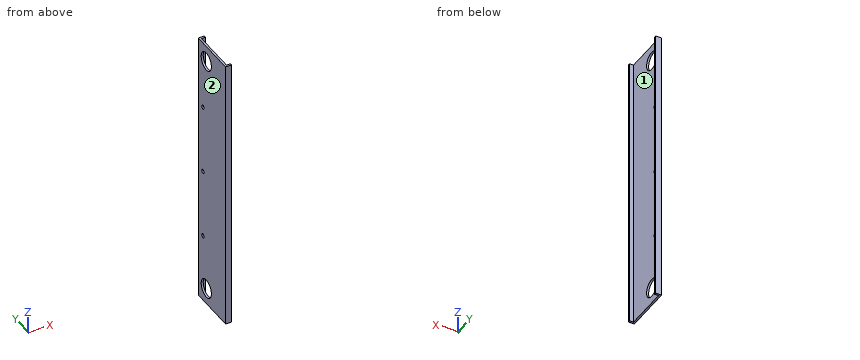
Autodesk Inventor part; units mm, degrees
ref_plane "YZ Plane" through (0, 0, 0) normal (1, 0, 0) x (0, 1, 0)
ref_plane "XZ Plane" through (0, 0, 0) normal (0, 1, 0) x (-1, 0, 0)
ref_plane "XY Plane" through (0, 0, 0) normal (0, 0, 1) x (1, 0, 0)
sketch "Sketch1" plane through (0, 0, 0) normal (0, 0, 1) x (1, 0, 0)
  line L0 (0, 0) -> (9.525, 0)
  line L1 (9.525, 76.2) -> (0, 76.2)
  line L2 (0, 76.2) -> (0, 0)
  line L3 (9.525, 3.175) -> (3.175, 3.175)
  line L4 (3.175, 3.175) -> (3.175, 73.025)
  line L5 (3.175, 73.025) -> (9.525, 73.025)
  line L6 (9.525, 0) -> (9.525, 3.175)
  line L7 (9.525, 73.025) -> (9.525, 76.2)
  dimension "d0" = 3.175
  dimension "d2" = 3.175
  dimension "d3" = 3.175
  dimension "d4" = 76.2
  dimension "d5" = 9.525
extrude "Extrusion1" add sketch "Sketch1" along normal blind 434.975
sketch "Sketch2" plane through (3.175, 3.175, 0) normal (1, 0, 0) x (0, 0, -1)
  line L0 (0, 0) -> (0, 69.85)
  line L1 (0, 73.025) -> (-434.975, 73.025)
  line L2 (0, -3.175) -> (-434.975, -3.175)
  line L3 (-434.975, 0) -> (-434.975, -3.175)
  line L4 (-434.975, 73.025) -> (-434.975, 69.85)
  line L5 (0, 69.85) -> (0, 73.025)
  line L6 (0, -3.175) -> (0, 0)
  circle A0 centre (-25.4, 50.8) radius 14.2875
  line L7 (-434.975, 69.85) -> (-434.975, 0)
  circle A1 centre (-409.575, 50.8) radius 14.2875
  circle A2 centre (-217.4875, 60.325) radius 3.175
  circle A3 centre (-326.2313, 60.325) radius 3.175
  circle A4 centre (-108.7438, 60.325) radius 3.175
  dimension "d8" = 28.575
  dimension "d10" = 53.975
  dimension "d11" = 25.4
  dimension "d14" = 25.4
  dimension "d15" = 53.975
  dimension "d16" = 28.575
  dimension "d17" = 6.35
  dimension "d18" = 12.7
  dimension "d19" = 217.4875
  dimension "d20" = 108.7438
  dimension "d21" = 108.7438
  dimension "d22" = 6.35
  dimension "d23" = 6.35
  dimension "d24" = 434.975
extrude "Extrusion2" cut sketch "Sketch2" against normal blind 508 contours A0 | A1 | A2 | A3 | A4
equation "\"d3\" = d2"
equation "\"d14\" = d11"
equation "\"d15\" = d10"
equation "\"d16\" = d8"
equation "\"d19\" = 0.5 * d24"
equation "\"d20\" = d21"
equation "\"d21\" = 0.5 * d19"
equation "\"d22\" = d17"
equation "\"d23\" = d17"
properties part number "uptake bearing plate"
Geometry: final body of the model. Coordinates: model frame, mm. Face numbers are marked on the shaded views. Round coordinates to 2 decimals unless told otherwise and drop trailing zeros. Write each loop counter-clockwise with the first axis right and the second up, starting at its lowest first coordinate (ties: lowest second). Pieces come first, ordered by that corner, then holes.
Item 1: Pin query (flat end, axial travel): P1, Ø5.5, axis at y = 63.5, z = 217.49, coming from the -X side; P2, Ø10, axis at y = 55.5, z = 336, coming from the +X side (3 decimals); P3, Ø4, axis at x = 5.5, z = 197.5, coming from the -Y side. Return the tip coordinate at first contact, or that it passes through.
Item 2: Section query B-B (z = 388). Return loops of the section in (x, y) (3 decimals), plus the area to 3 significant figures.
Item 3: Material intervals for L1, parallel to Z at x = 1.75, y = 52.5 (3 decimals); L2, parallel to Y at x = 5.5, z = 357.5 (3 decimals); L3, parallel to Z at x = 1, y = 63 (3 decimals), sorted ascending.
Item 4: Section query C-C (y = 11.5). Return loops of the section in (x, z) (3 decimals), plus the area to 3 significant figures.
Item 5: Section query A-A (z = 25.4). Return loops of the section in (x, y) (1 decimal), plus the area to 3 significant figures.
Item 6: Mould query, pull axis Y, two halves, no side actions, for the marked faces 1 and 2. Classes: +Y half, -Y half, draft (parallel to the pull), parting line (faces both ways), or undercut.
Completed:
1. P1: passes through
1. P2: stops at x = 3.175
1. P3: stops at y = 0
2. outline: (0, 0) - (9.525, 0) - (9.525, 3.175) - (3.175, 3.175) - (3.175, 73.025) - (9.525, 73.025) - (9.525, 76.2) - (0, 76.2) - close
2. area: 282 mm2
3. L1: z = 0 to 11.189, 39.611 to 395.364, 423.786 to 434.975
3. L2: y = 0 to 3.175, 73.025 to 76.2
3. L3: z = 0 to 14.324, 36.476 to 105.608, 111.879 to 214.352, 220.623 to 323.096, 329.367 to 398.499, 420.651 to 434.975
4. outline: (0, 0) - (3.175, 0) - (3.175, 434.975) - (0, 434.975) - close
4. area: 1,380 mm2
5. outline: (0, 0) - (9.5, 0) - (9.5, 3.2) - (3.2, 3.2) - (3.2, 39.7) - (0, 39.7) - close; (0, 68.3) - (3.2, 68.3) - (3.2, 73) - (9.5, 73) - (9.5, 76.2) - (0, 76.2) - close
5. area: 192 mm2
6. face 1: undercut
6. face 2: draft
